from build123d import *

# Parameters (mm, degrees)
F0_R     = 2.2479
F0_W     = 3.175
F0_H     = 19.05
F0_R_2   = 3.4925
F1_DEPTH = 6.35


with BuildPart() as f1:
    # F0 (on Top) → F1 (new body)
    with BuildSketch(Plane.XY):
        Polygon((203.2, -25.4), (203.2, 25.4), (-203.2, 25.4), (-203.2, -25.4), (-60.331323, -25.4), (-42.008828, -25.4), (40.984878, -25.4), (59.307373, -25.4), align=None)
        with Locations((-195.2625, -19.05)):
            Circle(F0_R, mode=Mode.SUBTRACT)
        with Locations((-195.2625, 0)):
            Rectangle(F0_W, F0_H, mode=Mode.SUBTRACT)
        with Locations((-139.7, 0)):
            Circle(F0_R_2, mode=Mode.SUBTRACT)
        with Locations((-195.2625, 19.05)):
            Circle(F0_R, mode=Mode.SUBTRACT)
        with Locations((-88.9, 0)):
            Circle(F0_R_2, mode=Mode.SUBTRACT)
        with Locations((-25.4, 0)):
            Circle(F0_R_2, mode=Mode.SUBTRACT)
        with Locations((195.2625, -19.05)):
            Circle(F0_R, mode=Mode.SUBTRACT)
        with Locations((88.9, 0)):
            Circle(F0_R_2, mode=Mode.SUBTRACT)
        with Locations((139.7, 0)):
            Circle(F0_R_2, mode=Mode.SUBTRACT)
        with Locations((195.2625, 0)):
            Rectangle(F0_W, F0_H, mode=Mode.SUBTRACT)
        with Locations((195.2625, 19.05)):
            Circle(F0_R, mode=Mode.SUBTRACT)
        with BuildLine():
            Line((59.307373, -88.9), (59.307373, -25.4))
            Line((59.307373, -25.4), (40.984878, -25.4))
            Line((40.984878, -25.4), (40.984878, -88.9))
            ThreePointArc((40.984878, -88.9), (50.146126, -94.667148), (59.307373, -88.9))
        make_face()
        with BuildLine():
            Line((-42.008828, -25.4), (-60.331323, -25.4))
            Line((-60.331323, -25.4), (-60.331323, -88.9))
            ThreePointArc((-60.331323, -88.9), (-51.170076, -94.667148), (-42.008828, -88.9))
            Line((-42.008828, -88.9), (-42.008828, -25.4))
        make_face()
    extrude(amount=F1_DEPTH)


solid = f1.part
Can you work these out from the model? Positions are in its coordinate system, mm. Give positions to 0.01 mm unless a question says otherwise; leave off trailing zeros. Loops run counter-clockwise (first coordinate to the right, second up) from the corner with the lowest first, then second, coordinate; pieces in that order, holes last. Notation, with made-up numbers: (-19.5, 10.25) - (16.5, 10.25) arc R11 cw to (16.5, 15.25) - close; hole circle Ø2 at (40, 2.25). An arc over 180 degrees is marked (long way). Answer as a JSON object with one key per item and string values.
Q1. Imagine slicing it at B-B on x = -25.4. Write out the boundary of the cut face in (y, z), plus the area to 3 significant figures.
Geometry says:
{"outline": "(-25.4, 0) - (-3.49, 0) - (-3.49, 6.35) - (-25.4, 6.35) - close; (3.49, 0) - (25.4, 0) - (25.4, 6.35) - (3.49, 6.35) - close", "area": "278 mm²"}
Q2. If we mould it in two halves opening along Y, with no side actions, what happens to faces 1 (the cylindrical face through (-28.89, 0.15, 3.13)), 2 (the flat face through (-3, -7, 0)), 3 (the cylindrical face through (92.23, 1.05, 3.13))? For each: pulls with the +Y half, pulls with the -Y half, needs draft (parallel to the pull), parting line crosses it, or undercut.
Geometry says:
{"face 1": "undercut", "face 2": "needs draft", "face 3": "undercut"}
Q3. Imagine slicing it at C-C on y = -53. Write out the boundary of the cut face in (x, z), plus the area to 3 significant figures.
Geometry says:
{"outline": "(-60.33, 0) - (-42.01, 0) - (-42.01, 6.35) - (-60.33, 6.35) - close; (40.98, 0) - (59.31, 0) - (59.31, 6.35) - (40.98, 6.35) - close", "area": "233 mm²"}
Q4. If I drill on L1, parallel to X at y = -48.5, z = 4.75; L2, parallel to Y at x = -139.7, z = 5.25; L3, parallel to Y at x = 148.5, z = 5.5, over which ranges is the centre line in solid material (lowest first)?
Geometry says:
{"L1": "-60.33 to -42.01, 40.98 to 59.31", "L2": "-25.4 to -3.49, 3.49 to 25.4", "L3": "-25.4 to 25.4"}
Q5. Imagine slicing it at A-A on y = 0. Give the number of separate pieces and of enclosed holes in the cut face, plus the area to 3 significant figures.
Geometry says:
{"separate pieces": "8", "enclosed holes": "0", "area": "2,320 mm²"}
Q6. Will these pins go through, and if not, where does the flat tip stop? P1, Ø1.9, axis at y = -49, z = 3.5, coming from the -X side; P2, Ø2, axis at y = -38, z = 5, coming from the +X side; P3, Ø1, axis at x = -130.5, z = 2, coming from the -Y side; P4, Ø3.5, axis at x = 195.26, y = -19.05, coming from the -Z side.
Geometry says:
{"P1": "x = -60.33", "P2": "x = 59.31", "P3": "y = -25.4", "P4": "through"}
